Build history of the part. All positions in model axes, mm. A direction names the side the tool comes from. Round coordinates to 2 decimals unless told otherwise and drop trailing zeros. Order: outer loops, then holes, each group sorted by start corner. A loop starts at its lowest first (then second) coordinate and runs counter-clockwise, first axis right, second up. Notation, with made-up numbers: (-0.5, 3) -> (17.5, 3) arc R25 ccw to (17.5, 16) -> close; hole circle Ø1 at (-28.5, 43). An arc over 180 degrees is marked (long way). Write item = value, one per line.
from build123d import *

# Parameters (mm, degrees)
F0_R     = 7
F1_DEPTH = 2
F2_R     = 5
F2_R_2   = 4
F3_DEPTH = 14
F4_SIZE  = 0.49999


# Not quite as in the source:
# - a fillet or chamfer is up to 0.001 mm smaller than in the source, because OpenCascade refuses the exact size


with BuildPart() as f1:
    # F0 (on Top) → F1 (new body)
    with BuildSketch(Plane.XY):
        Circle(F0_R)
    extrude(amount=F1_DEPTH)

    # F2 (on face) → F3 (join)
    with BuildSketch(Plane.XY.offset(2)):
        Circle(F2_R)
        Circle(F2_R_2, mode=Mode.SUBTRACT)
    extrude(amount=F3_DEPTH)

    # F4 (size 0.5 in the source; OpenCascade refuses exactly that, so slightly less here)
    f4_edges = [f1.edges().sort_by_distance(p)[0] for p in [
        (-5, 0, 16),
        (-4, 0, 16),
    ]]
    chamfer(f4_edges, length=F4_SIZE)


solid = f1.part
Q1. Which spindle directions (+Z, -Z, +X, -X, +Y, -Y) get a long thin tool onto all of the face, cutting with end or side? Do faces 4 (the face through (6.466, -2.681, 0.986)), 5 (the face through (-2, 5, 2)). Say none if no direction does.
Check values:
face_4 = +Z, -Z
face_5 = +Z
Q2. Mould opens along X. For faces 1 (the face through (-0.867, -3.905, 8.656)), 2 (the face through (-1.08, -4.88, 8.66)), 3 (the face through (0, 0, 0)) say: released by +X, released by -X, zero draft, split by the parting line, or undercut.
Check values:
face_1 = undercut
face_2 = split by the parting line
face_3 = zero draft
Q3. Probe probe 1 along Y at (x, z) = (0, 6.75); probe 2 along Z at (x, y) = (-5.75, 3.25); probe 3 along X at (y, z) = (2, 3.75). List the from-to ranges inside material, lowest first.
Check values:
probe_1 = -5 to -4, 4 to 5
probe_2 = 0 to 2
probe_3 = -4.58 to -3.46, 3.46 to 4.58
Q4. Cut at D-D, the plane y = 5.75. List the corners of the cut face in (x, z), and give its area (3 significant figures).
Check values:
outline = (-3.99, 0) -> (3.99, 0) -> (3.99, 2) -> (-3.99, 2) -> close
area = 16.0 mm²
Q5. Flat gauge pins, fed straight in: pin 1 (6 mm diameter, centred on x = 4.5, z = 5.5, fed in from -Y); pin 2 (3 mm diameter, centred on y = -3, z = 5, fed in from -X); pin 3 (4 mm diameter, centred on x = 3.5, z = 2, fed in from +Y). Where does each tip first touch, or does it go through?
Check values:
pin_1 = -4.77
pin_2 = -4.77
pin_3 = 6.84
Q6. Cut at C-C, the plane z = 12.5. List the corners of the cut face in (x, y), and give its area (3 significant figures).
Check values:
outline = circle Ø10 at (0, 0); hole circle Ø8 at (0, 0)
area = 28.3 mm²
